from build123d import *

# Parameters (mm, degrees)
SKETCH1_W           = 170.58
SKETCH1_H           = 69.88
BOSS_EXTRUDE1_DEPTH = 5
SKETCH6_R           = 1.25
CUT_EXTRUDE2_DEPTH  = 8
SKETCH7_R           = 1.75
CUT_EXTRUDE3_DEPTH  = 8
BOSS_EXTRUDE2_DEPTH = 25
SKETCH9_R           = 1.75
SKETCH9_R_2         = 1.749999999
CUT_EXTRUDE4_DEPTH  = 10
CUT_EXTRUDE5_DEPTH  = 10
SKETCH11_R          = 2.5
CUT_EXTRUDE6_DEPTH  = 10


with BuildPart() as part:
    # Sketch1 → Boss-Extrude1 (new body)
    with BuildSketch(Plane(origin=(0, 0, 0), x_dir=(1, 0, 0), z_dir=(0, 1, 0))):
        with Locations((12.23073352, -487.847955707)):
            Rectangle(SKETCH1_W, SKETCH1_H)
    extrude(amount=BOSS_EXTRUDE1_DEPTH)

    # Sketch6 → Cut-Extrude2 (cut)
    with BuildSketch(Plane(origin=(0, 5, 0), x_dir=(1, 0, 0), z_dir=(0, 1, 0))):
        with Locations(Location((-30.70426648, -483.202955707, 0), (0, 0, 270))):
            Circle(SKETCH6_R)
        with Locations(Location((-23.20426648, -490.702955707, 0), (0, 0, 270))):
            Circle(SKETCH6_R)
        with Locations(Location((-30.70426648, -498.202955707, 0), (0, 0, 270))):
            Circle(SKETCH6_R)
        with Locations(Location((-38.20426648, -490.702955707, 0), (0, 0, 270))):
            Circle(SKETCH6_R)
        with Locations(Location((-38.20426648, -487.202955707, 0), (0, 0, 270))):
            Circle(SKETCH6_R)
        with Locations(Location((-38.20426648, -494.202955707, 0), (0, 0, 270))):
            Circle(SKETCH6_R)
        with Locations(Location((-23.20426648, -487.202955707, 0), (0, 0, 270))):
            Circle(SKETCH6_R)
        with Locations(Location((-23.20426648, -494.202955707, 0), (0, 0, 270))):
            Circle(SKETCH6_R)
        with Locations(Location((-27.20426648, -498.202955707, 0), (0, 0, 270))):
            Circle(SKETCH6_R)
        with Locations(Location((-34.20426648, -498.202955707, 0), (0, 0, 270))):
            Circle(SKETCH6_R)
        with Locations(Location((-27.20426648, -483.202955707, 0), (0, 0, 270))):
            Circle(SKETCH6_R)
        with Locations(Location((-34.20426648, -483.202955707, 0), (0, 0, 270))):
            Circle(SKETCH6_R)
        with Locations(Location((55.69573352, -483.202955707, 0), (0, 0, 270))):
            Circle(SKETCH6_R)
        with Locations(Location((55.69573352, -498.202955707, 0), (0, 0, 270))):
            Circle(SKETCH6_R)
        with Locations(Location((63.19573352, -490.702955707, 0), (0, 0, 270))):
            Circle(SKETCH6_R)
        with Locations(Location((48.19573352, -490.702955707, 0), (0, 0, 270))):
            Circle(SKETCH6_R)
        with Locations(Location((59.19573352, -483.202955707, 0), (0, 0, 270))):
            Circle(SKETCH6_R)
        with Locations(Location((52.19573352, -483.202955707, 0), (0, 0, 270))):
            Circle(SKETCH6_R)
        with Locations(Location((48.19573352, -487.202955707, 0), (0, 0, 270))):
            Circle(SKETCH6_R)
        with Locations(Location((48.19573352, -494.202955707, 0), (0, 0, 270))):
            Circle(SKETCH6_R)
        with Locations(Location((59.19573352, -498.202955707, 0), (0, 0, 270))):
            Circle(SKETCH6_R)
        with Locations(Location((52.19573352, -498.202955707, 0), (0, 0, 270))):
            Circle(SKETCH6_R)
        with Locations(Location((63.19573352, -487.202955707, 0), (0, 0, 270))):
            Circle(SKETCH6_R)
        with Locations(Location((63.19573352, -494.202955707, 0), (0, 0, 270))):
            Circle(SKETCH6_R)
    extrude(amount=-CUT_EXTRUDE2_DEPTH, mode=Mode.SUBTRACT)

    # Sketch7 → Cut-Extrude3 (cut)
    with BuildSketch(Plane.XZ):
        with Locations(Location((12.49573352, 489.082955707, 0), (0, 0, 270))):
            Circle(SKETCH7_R)
        with Locations(Location((12.49573352, 501.552955707, 0), (0, 0, 270))):
            Circle(SKETCH7_R)
    extrude(amount=-CUT_EXTRUDE3_DEPTH, mode=Mode.SUBTRACT)

    # Sketch8 → Boss-Extrude2 (add)
    with BuildSketch(Plane(origin=(0, 5, 0), x_dir=(1, 0, 0), z_dir=(0, 1, 0))):
        Polygon((53.19573352, -471.967955707), (55.69573352, -471.967955707), (58.19573352, -471.967955707), (58.19573352, -468.967955707), (53.19573352, -468.967955707), align=None)
        Polygon((-33.20426648, -471.967955707), (-33.20426648, -468.967955707), (-30.70426648, -468.967955707), (-28.20426648, -468.967955707), (-28.20426648, -471.967955707), align=None)
        Polygon((-49.44426648, -493.202955707), (-49.44426648, -490.702955707), (-49.44426648, -488.202955707), (-52.44426648, -488.202955707), (-52.44426648, -493.202955707), align=None)
    extrude(amount=BOSS_EXTRUDE2_DEPTH)

    # Sketch9 → Cut-Extrude4 (cut)
    with BuildSketch(Plane(origin=(0, 5, 0), x_dir=(1, 0, 0), z_dir=(0, 1, 0))):
        with Locations(Location((12.49573352, -476.612955707, 0), (0, 0, 270))):
            Circle(SKETCH9_R)
        with Locations(Location((12.49573352, -464.142955707, 0), (0, 0, 270))):
            Circle(SKETCH9_R)
        with Locations(Location((-59.05926648, -506.787955707, 0), (0, 0, 270))):
            Circle(SKETCH9_R_2)
    extrude(amount=-CUT_EXTRUDE4_DEPTH, mode=Mode.SUBTRACT)

    # Sketch10 → Cut-Extrude5 (cut)
    with BuildSketch(Plane(origin=(0, 5, 0), x_dir=(1, 0, 0), z_dir=(0, 1, 0))):
        Polygon((-73.05926648, -522.787955707), (-73.05926648, -512.787955707), (-63.05926648, -522.787955707), align=None)
        Polygon((97.52073352, -522.787955707), (87.52073352, -522.787955707), (97.52073352, -512.787955707), align=None)
    extrude(amount=-CUT_EXTRUDE5_DEPTH, mode=Mode.SUBTRACT)

    # Sketch11 → Cut-Extrude6 (cut)
    with BuildSketch(Plane(origin=(0, 5, 0), x_dir=(1, 0, 0), z_dir=(0, 1, 0))):
        with Locations(Location((-30.70426648, -490.702955707, 0), (0, 0, 270))):
            Circle(SKETCH11_R)
        with Locations(Location((55.69573352, -490.702955707, 0), (0, 0, 270))):
            Circle(SKETCH11_R)
    extrude(amount=-CUT_EXTRUDE6_DEPTH, mode=Mode.SUBTRACT)


solid = part.part
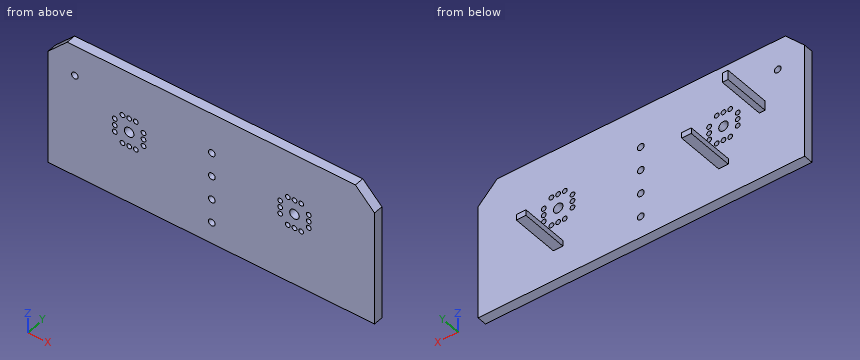
The model under review builds one solid part; all positions refer to its coordinate system, in mm. Round coordinates to 2 decimals unless told otherwise and drop trailing zeros. Write each loop counter-clockwise with the first axis right and the second up, starting at its lowest first coordinate (ties: lowest second). Pieces come first, ordered by that corner, then holes. Notation, with made-up numbers: (33.25, 88) - (73.25, 88) arc R19 ccw to (73.25, 106) - close; hole circle Ø6 at (10.25, 53.5). An arc over 180 degrees is marked (long way). One line per item, written item: value. Start each with the question number.
1. Consider section A-A on y = 21.5. Write out the cut boundary in (x, z), and give its area (3 significant figures).
2. Consider section B-B on z = 510.5. Write out the cut boundary in (x, y).
3. Consider section C-C on x = 32. Write out the cut boundary in (y, z), and give its area (3 significant figures).
4. To check wall thickness, follow L1, parallel to X at y = 4.75, z = 494; L2, parallel to Y at x = 24, z = 484.5; L3, parallel to X at y = 23.75, z = 490. State the ranges of each line that lie inside material, in increasing order. Write a range as from..to.
5. Consider section D-D on y = 3. State how many separate pieces and enclosed holes the cut face has, and give its area (3 significant figures).
6. Clearance check with flat-ended pins moving along their axes: P1, Ø3.5, axis at y = 14.5, z = 470.5, coming from the +X side; P2, Ø4, axis at x = 56.5, y = 12, coming from the +Z side; P3, Ø1.5, axis at x = -14.5, z = 497.5, coming from the +Y side. State where each tip first meets the part, or that it passes through.
Checks:
1. outline: (-52.44, 488.2) - (-49.44, 488.2) - (-49.44, 493.2) - (-52.44, 493.2) - close; (-33.2, 468.97) - (-28.2, 468.97) - (-28.2, 471.97) - (-33.2, 471.97) - close; (53.2, 468.97) - (58.2, 468.97) - (58.2, 471.97) - (53.2, 471.97) - close
1. area: 45.0 mm^2
2. outline: (-73.06, 0) - (97.52, 0) - (97.52, 5) - (-73.06, 5) - close
3. outline: (0, 452.91) - (5, 452.91) - (5, 522.79) - (0, 522.79) - close
3. area: 349 mm^2
4. L1: x = -73.06..-39.44, -36.97..-24.44, -21.97..46.96, 49.43..61.96, 64.43..97.52
4. L2: y = 0..5
4. L3: x = -52.44..-49.44
5. separate pieces: 1
5. enclosed holes: 31
5. area: 11,600 mm^2
6. P1: stops at x = 58.2
6. P2: stops at z = 471.97
6. P3: stops at y = 5
